Autodesk Inventor part; units mm, degrees
ref_plane "YZ Plane" through (0, 0, 0) normal (1, 0, 0) x (0, 1, 0)
ref_plane "XZ Plane" through (0, 0, 0) normal (0, 1, 0) x (-1, 0, 0)
ref_plane "XY Plane" through (0, 0, 0) normal (0, 0, 1) x (1, 0, 0)
sketch "スケッチ1" plane through (0, 0, 0) normal (0, 1, 0) x (-1, 0, 0)
  circle A0 centre (0, 0) radius 35
  circle A1 centre (0, 0) radius 40
  dimension "d0" = 70
  dimension "d1" = 80
extrude "押し出し1" add sketch "スケッチ1" along normal blind 80
sketch "スケッチ2" plane through (0, 0, 0) normal (0, -1, 0) x (1, 0, 0)
  line L0 (37.5, 1.6) -> (-37.5, 1.6)
  line L1 (-37.5, 1.6) -> (-37.5, -1.6)
  line L2 (-37.5, -1.6) -> (37.5, -1.6)
  line L3 (37.5, -1.6) -> (37.5, 1.6)
  line L4 (37.5, 1.6) -> (-37.5, -1.6) construction
  line L5 (-37.5, 1.6) -> (37.5, -1.6) construction
  line L6 (-1.6, 37.5) -> (1.6, 37.5)
  line L7 (1.6, 37.5) -> (1.6, -37.5)
  line L8 (1.6, -37.5) -> (-1.6, -37.5)
  line L9 (-1.6, -37.5) -> (-1.6, 37.5)
  line L10 (-1.6, 37.5) -> (1.6, -37.5) construction
  line L11 (1.6, 37.5) -> (-1.6, -37.5) construction
  line L12 (3.6, 38.6) -> (-3.6, 38.6)
  line L13 (-3.6, 38.6) -> (-3.6, 36.4)
  line L14 (-3.6, 36.4) -> (3.6, 36.4)
  line L15 (3.6, 36.4) -> (3.6, 38.6)
  line L16 (3.6, 38.6) -> (-3.6, 36.4) construction
  line L17 (-3.6, 38.6) -> (3.6, 36.4) construction
  line L18 (3.6, -36.4) -> (-3.6, -36.4)
  line L19 (-3.6, -36.4) -> (-3.6, -38.6)
  line L20 (-3.6, -38.6) -> (3.6, -38.6)
  line L21 (3.6, -38.6) -> (3.6, -36.4)
  line L22 (3.6, -36.4) -> (-3.6, -38.6) construction
  line L23 (-3.6, -36.4) -> (3.6, -38.6) construction
  line L24 (36.4, 3.6) -> (38.6, 3.6)
  line L25 (38.6, 3.6) -> (38.6, -3.6)
  line L26 (38.6, -3.6) -> (36.4, -3.6)
  line L27 (36.4, -3.6) -> (36.4, 3.6)
  line L28 (36.4, 3.6) -> (38.6, -3.6) construction
  line L29 (38.6, 3.6) -> (36.4, -3.6) construction
  line L30 (-36.4, 3.6) -> (-38.6, 3.6)
  line L31 (-38.6, 3.6) -> (-38.6, -3.6)
  line L32 (-38.6, -3.6) -> (-36.4, -3.6)
  line L33 (-36.4, -3.6) -> (-36.4, 3.6)
  line L34 (-36.4, 3.6) -> (-38.6, -3.6) construction
  line L35 (-38.6, 3.6) -> (-36.4, -3.6) construction
  point P0 (0, 0)
  point P1 (0, 37.5)
  point P2 (0, -37.5)
  point P3 (37.5, 0)
  point P4 (-37.5, 0)
  dimension "d4" = 75
  dimension "d5" = 3.2
  dimension "d6" = 3.2
  dimension "d7" = 75
  dimension "d8" = 7.2
  dimension "d9" = 2.2
  dimension "d10" = 7.2
  dimension "d11" = 2.2
  dimension "d12" = 2.2
  dimension "d13" = 7.2
  dimension "d14" = 2.2
  dimension "d15" = 7.2
extrude "押し出し2" cut sketch "スケッチ2" against normal blind 80
sketch "スケッチ3" plane through (0, 0, 0) normal (0, -1, 0) x (1, 0, 0)
  circle A0 centre (0, 0) radius 40
extrude "押し出し3" add sketch "スケッチ3" along normal blind 3
properties part number "box"
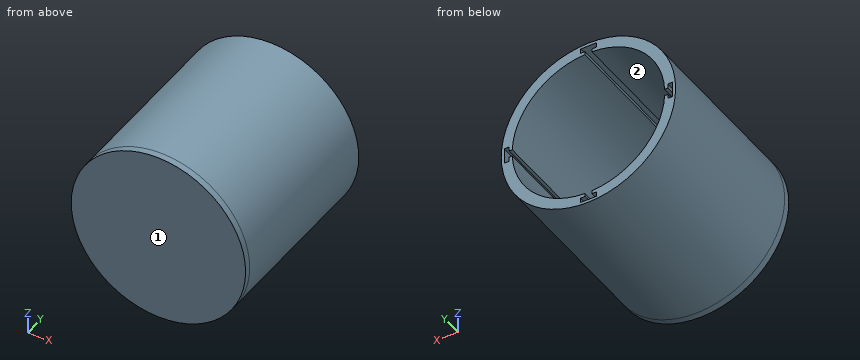
Read the model definition and answer for the solid it produces. Units are mm, in the model's axes. Face numbers are marked on the shaded views. Give positions to 0.01 mm unless a question says otherwise; leave off trailing zeros. Write each loop counter-clockwise with the first axis right and the second up, starting at its lowest first coordinate (ties: lowest second). Pieces come first, ordered by that corner, then holes. Notation, with made-up numbers: (-17.5, 63.5) -> (32.5, 63.5) arc R20 ccw to (32.5, 78.5) -> close; hole circle Ø6 at (-39.75, 21). An arc over 180 degrees is marked (long way). Answer as a JSON object with one key per item and string values. Group by question number.
1) Consider L1, parallel to Z at x = 0, y = 71; L2, parallel to Y at x = 33, z = -3.5; L3, parallel to Z at x = 22, y = 45. Determine where each line is inside the solid, lowest interval first. Write a range as from..to.
2) Find section C-C (x = 0). Write down the section's boundary in (y, z).
3) The mould has two halves that part along X. Classify the marked faces 1 and 2: +X half, -X half, draft (parallel to the pull), parting line (faces both ways), or undercut.
4) Each of these flat-tipped pins is pushed along its axis until it touches: P1, Ø2, axis at y = 26, z = 5, coming from the -X side; P2, Ø1.1, axis at y = 27, z = 37.5, coming from the -X side; P3, Ø12, axis at x = -30, y = 53.5, coming from the +Z side. Where does it stop, or does it pass through?
5) Find section B-B (z = 0). Write down the section's boundary in (x, y).
Values follow:
{
 "1": {"L1": "z = -40..-38.6, 38.6..40", "L2": "y = -3..0", "L3": "z = -33.41..-27.22, 27.22..33.41"},
 "2": {"outline": "(-3, -40) -> (80, -40) -> (80, -38.6) -> (0, -38.6) -> (0, 38.6) -> (80, 38.6) -> (80, 40) -> (-3, 40) -> close"},
 "3": {"face 1": "draft", "face 2": "undercut"},
 "4": {"P1": "stops at x = -39.8", "P2": "stops at x = -15.32", "P3": "stops at z = 32"},
 "5": {"outline": "(-40, -3) -> (40, -3) -> (40, 80) -> (38.6, 80) -> (38.6, 0) -> (-38.6, 0) -> (-38.6, 80) -> (-40, 80) -> close"}
}
